Autodesk Inventor part; units mm, degrees
ref_plane "YZ Plane" through (0, 0, 0) normal (1, 0, 0) x (0, 1, 0)
ref_plane "XZ Plane" through (0, 0, 0) normal (0, 1, 0) x (-1, 0, 0)
ref_plane "XY Plane" through (0, 0, 0) normal (0, 0, 1) x (1, 0, 0)
sketch "Sketch1" plane through (0, 0, 0) normal (0, 1, 0) x (-1, 0, 0)
  line L0 (-75, 40) -> (75, 40)
  line L1 (75, 40) -> (75, -40)
  line L2 (75, -40) -> (-75, -40)
  line L3 (-75, -40) -> (-75, 40)
  line L4 (-75, 40) -> (75, -40) construction
  line L5 (75, 40) -> (-75, -40) construction
  point P0 (0, 0)
  dimension "d0" = 150
  dimension "d1" = 80
extrude "Extrusion1" add sketch "Sketch1" along normal blind 3
sketch "Sketch4" plane through (0, 3, 0) normal (0, 1, 0) x (1, 0, 0)
  line L0 (75, 40) -> (-75, 40)
  line L1 (-10, 40) -> (10, 40)
  line L2 (10, 40) -> (10, 20)
  line L3 (-10, 40) -> (-10, 20)
  line L4 (-10, 20) -> (10, 20)
  line L5 (-13, 40) -> (-7, 40)
  line L6 (7, 40) -> (13, 40)
  line L7 (-10, 40) -> (-10, 35)
  line L8 (10, 40) -> (10, 35)
  line L9 (-10, 35) -> (-10, 32)
  line L10 (10, 35) -> (10, 32)
  line L11 (-10, 20) -> (-10, 23)
  line L12 (10, 20) -> (10, 23)
  circle A0 centre (-10, 23) radius 3
  circle A1 centre (10, 23) radius 3
  circle A2 centre (-10, 32) radius 3
  circle A3 centre (10, 32) radius 3
  line L13 (-13, 32) -> (-13, 23)
  line L14 (-7, 32) -> (-7, 23)
  line L15 (7, 32) -> (7, 23)
  line L16 (13, 32) -> (13, 23)
  line L17 (-10, 20) -> (-7, 20)
  line L18 (-7, 20) -> (-7, 40)
  line L19 (-7, 40) -> (-10, 40)
  line L20 (-10, 40) -> (-10, 20)
  line L21 (-10, 40) -> (-13, 40)
  line L22 (-13, 40) -> (-13, 20)
  line L23 (-13, 20) -> (-10, 20)
  line L24 (-10, 20) -> (-10, 40)
  line L25 (10, 20) -> (7, 20)
  line L26 (7, 20) -> (7, 40)
  line L27 (7, 40) -> (10, 40)
  line L28 (10, 40) -> (10, 20)
  line L29 (10, 20) -> (13, 20)
  line L30 (13, 20) -> (13, 40)
  line L31 (13, 40) -> (10, 40)
  line L32 (10, 40) -> (10, 20)
  point P0 (0, 0)
  point P1 (0, 40)
  point P2 (7, 40)
  point P3 (7, 32)
  point P4 (-7, 40)
  point P5 (-13, 40)
  dimension "d14" = 20
  dimension "d15" = 20
  dimension "d16" = 6
  dimension "d17" = 6
  dimension "d18" = 5
  dimension "d19" = 5
  dimension "d20" = 3
  dimension "d21" = 3
  dimension "d22" = 3
  dimension "d23" = 3
extrude "Extrusion3" cut sketch "Sketch4" against normal through all contours A3 L2 | L16 A1 L2 A3 | L2 A3 | L2 A1 L15 A3 | A1 L2 | L2 A1 | A2 L3 | L14 A0 L3 A2 | L3 A2 | L3 A0 L13 A2 | A0 L3 | L3 A0
sketch "Sketch5" plane through (0, 3, 0) normal (0, 1, 0) x (1, 0, 0)
  line L0 (-75, 40) -> (-75, -40)
  line L1 (75, 40) -> (-75, 40)
  line L2 (-75, 40) -> (-75, 15)
  line L3 (-75, 15) -> (75, 15)
  line L4 (75, 15) -> (75, 40)
  line L5 (21.6, 15) -> (-21.6, 15)
  line L6 (75, 15) -> (31.8, 15)
  line L7 (31.8, 15) -> (31.8, -28.2)
  line L8 (31.8, -28.2) -> (75, -28.2)
  line L9 (75, -28.2) -> (75, 15)
  line L10 (31.8, 15) -> (75, -28.2)
  line L11 (75, 15) -> (31.8, -28.2)
  circle A0 centre (53.4, -6.6) radius 11
  line L12 (37.9, -22.1) -> (68.9, -22.1)
  line L13 (68.9, -22.1) -> (68.9, 8.9)
  line L14 (68.9, 8.9) -> (37.9, 8.9)
  line L15 (37.9, 8.9) -> (37.9, -22.1)
  line L16 (37.9, -22.1) -> (68.9, 8.9) construction
  line L17 (68.9, -22.1) -> (37.9, 8.9) construction
  circle A1 centre (37.9, 8.9) radius 2
  circle A2 centre (68.9, 8.9) radius 2
  circle A3 centre (68.9, -22.1) radius 2
  circle A4 centre (37.9, -22.1) radius 2
  point P0 (309.988, -32.2194)
  dimension "d26" = 25
  dimension "d49" = 150
  dimension "d50" = 43.2
  dimension "d51" = 43.2
  dimension "d52" = 22
  dimension "d53" = 31
  dimension "d54" = 31
  dimension "d55" = 4
  dimension "d56" = 4
  dimension "d57" = 4
  dimension "d58" = 4
extrude "Extrusion4" cut sketch "Sketch5" against normal through all contours A2 L13 L11 | L11 L14 A2 | A1 L14 L10 | L10 L15 A1 | A3 L12 L10 | L10 L13 A3 | L13 A2 L11 | L11 A2 L14 | A4 L15 L11 | L11 L12 A4 | L14 A1 L10 | L10 A1 L15 | L12 A3 L10 | L10 A3 L13 | L15 A4 L11 | L11 A4 L12 | A0 L10 L11 | L11 L10 A0 | L10 L11 A0 | A0 L11 L10
extrude "Extrusion5" cut sketch "Sketch4" against normal blind 1.2 contours L30 A3 L2 L0 | L2 A3 L26 L0 | L18 A2 L3 L0 | L3 A2 L22 L0
sketch "Sketch6" plane through (0, 3, 0) normal (0, 1, 0) x (1, 0, 0)
  line L0 (75, 40) -> (-75, 40)
  line L1 (0, 40) -> (0, 15)
  line L2 (0, 15) -> (0, -28.2)
  line L3 (-21.6, 15) -> (21.6, 15)
  line L4 (21.6, 15) -> (21.6, -28.2)
  line L5 (21.6, -28.2) -> (-21.6, -28.2)
  line L6 (-21.6, -28.2) -> (-21.6, 15)
  line L7 (-21.6, 15) -> (21.6, -28.2) construction
  line L8 (21.6, 15) -> (-21.6, -28.2) construction
  circle A0 centre (0, -6.6) radius 5.1
  line L9 (0, 15) -> (75, 15)
  line L10 (75, 15) -> (31.8, 15)
  line L11 (31.8, 15) -> (31.8, -6.6)
  line L12 (31.8, -6.6) -> (53.4, -6.6)
  line L13 (53.4, -6.6) -> (0, -6.6)
  line L14 (0, -6.6) -> (-53.4, -6.6)
  circle A1 centre (-53.4, -6.6) radius 5.1
  line L15 (0, -25.6) -> (0, 12.4)
  circle A2 centre (0, 12.4) radius 2.5
  line L16 (0, 12.4) -> (0, 10.4)
  circle A3 centre (0, 10.4) radius 2.5
  circle A4 centre (0, -25.6) radius 2.5
  line L17 (0, -25.6) -> (0, -23.6)
  circle A5 centre (0, -23.6) radius 2.5
  line L18 (-2.5, -23.6) -> (-2.5, -25.6)
  line L19 (2.5, -23.6) -> (2.5, -25.6)
  line L20 (-2.5, 12.4) -> (-2.5, 10.4)
  line L21 (2.5, 12.4) -> (2.5, 10.4)
  line L22 (-53.4, 9.4) -> (-53.4, -22.6)
  circle A6 centre (-53.4, -22.6) radius 3
  circle A7 centre (-53.4, 9.4) radius 3
  point P0 (0, 0)
  dimension "d59" = 25
  dimension "d60" = 43.2
  dimension "d61" = 43.2
  dimension "d62" = 43.2
  dimension "d63" = 10.2
  dimension "d64" = 43.2
  dimension "d65" = 53.4
  dimension "d66" = 10.2
  dimension "d69" = 38
  dimension "d70" = 5
  dimension "d71" = 2
  dimension "d72" = 5
  dimension "d73" = 5
  dimension "d74" = 2
  dimension "d75" = 5
  dimension "d84" = 32
  dimension "d85" = 6
  dimension "d86" = 6
extrude "Extrusion6" cut sketch "Sketch6" against normal through all contours L2 A3 A2 | L2 A2 A3 | A3 A2 L2 | L2 A2 A3 | A2 A3 L2 | L2 A3 A2 | A2 L21 A3 | A3 L20 A2 | A6 | A7 | A1 L22 L14 | L14 L22 A1 | A0 L13 L2 | L2 L14 A0 | L13 A0 L2 | L2 A0 L14 | A5 A4 L2 | L2 A4 A5 | L22 A1 | A4 A5 L2 | L2 A5 A4 | L19 A4 A5 | A5 A4 L18 | A4 A5 L2 | L2 A5 A4
fillet "Fillet1" radius 20 4 edges at (75, 1.5, 40) (75, 1.5, -40) (-75, 1.5, 40) (-75, 1.5, -40)
sketch "Sketch7" plane through (0, 3, 0) normal (0, 1, 0) x (1, 0, 0)
  line L0 (0, 0) -> (22, 0)
  line L1 (22, 0) -> (22, -30)
  circle A0 centre (22, -30) radius 2
  line L2 (20, -30) -> (24, -30)
  line L3 (20, -30) -> (20, 0)
  line L4 (24, -30) -> (24, 0)
  line L5 (22, -30) -> (22, -10)
  circle A1 centre (22, -10) radius 2
  point P0 (24, -10)
  point P1 (20, -10)
  dimension "d90" = 4
  dimension "d88" = 22
  dimension "d89" = 30
  dimension "d91" = 20
extrude "Extrusion7" cut sketch "Sketch7" against normal through all contours A1 L1 A0 L3 | A1 L1 | A1 L1 | L2 A0 | A0 L1 L2 | A1 L4 A0 L1 | L2 L1 A0
properties part number "TopMount"
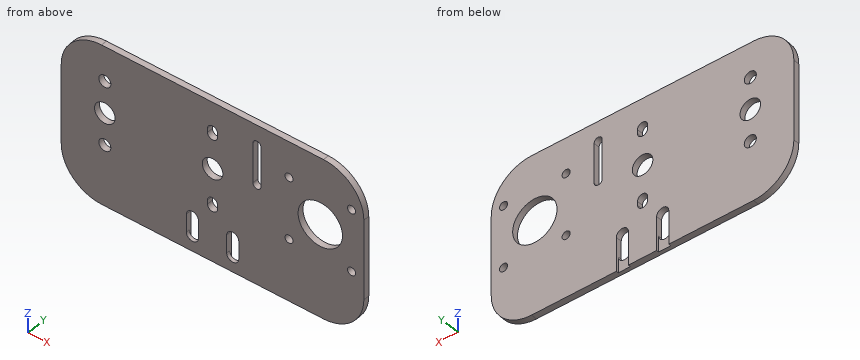
Read the model definition and answer for the solid it produces. Units are mm, in the model's axes. Round coordinates to 2 decimals unless told otherwise and drop trailing zeros. Write each loop counter-clockwise with the first axis right and the second up, starting at its lowest first coordinate (ties: lowest second). Pieces come first, ordered by that corner, then holes.
1. The part is cut by section C-C, the plane z = 6.6. Determine the outline of the cut face in (x, y).
2. The part is cut by section B-B, the plane x = -53.4. Determine the outline of the cut face in (y, z), then the cut area to 3 significant figures.
3. Given pin 1 Ø1.5 at (y, z) = (2, -29) entering from +X; pin 2 Ø3.5 at (x, z) = (-53.4, -9.4) entering from +Y; pin 3 Ø3 at (x, z) = (9.5, -36) entering from +Y; pin 4 Ø1 at (y, z) = (1, 24.5) entering from +X, each flat-ended and moving along its own axis, determine where each tip first touches the part or whether it passes through.
4. The part is cut by section A-A, the plane x = 53.4. Determine the outline of the cut face in (y, z), then the cut area to 3 significant figures.
5. Straight lines are drawn through the part: L1, parallel to Z at x = 37.9, y = 0.7; L2, parallel to Z at x = -53.4, y = 1.4; L3, parallel to X at y = 1, z = 6.6. For each, find the intervals that lie inside material, in ascending order.
6. The part is cut by section D-D, the plane x = -10. Determine the outline of the cut face in (y, z).
Values:
1. outline: (-75, 0) - (-58.5, 0) - (-58.5, 3) - (-75, 3) - close; (-48.3, 0) - (-5.1, 0) - (-5.1, 3) - (-48.3, 3) - close; (5.1, 0) - (42.4, 0) - (42.4, 3) - (5.1, 3) - close; (64.4, 0) - (75, 0) - (75, 3) - (64.4, 3) - close
2. outline: (0, -40) - (3, -40) - (3, -12.4) - (0, -12.4) - close; (0, -6.4) - (3, -6.4) - (3, 1.5) - (0, 1.5) - close; (0, 11.7) - (3, 11.7) - (3, 19.6) - (0, 19.6) - close; (0, 25.6) - (3, 25.6) - (3, 40) - (0, 40) - close
2. area: 173 mm2
3. pin 1: stops at x = 73.22
3. pin 2: passes through
3. pin 3: stops at y = 1.8
3. pin 4: stops at x = 74.6
4. outline: (0, -40) - (3, -40) - (3, -4.4) - (0, -4.4) - close; (0, 17.6) - (3, 17.6) - (3, 40) - (0, 40) - close
4. area: 174 mm2
5. L1: z = -40 to -10.9, -6.9 to 20.1, 24.1 to 40
5. L2: z = -40 to -12.4, -6.4 to 1.5, 11.7 to 19.6, 25.6 to 40
5. L3: x = -75 to -58.5, -48.3 to -5.1, 5.1 to 42.4, 64.4 to 75
6. outline: (0, -40) - (1.8, -40) - (1.8, -35) - (0, -35) - close; (0, -20) - (3, -20) - (3, 40) - (0, 40) - close
